from build123d import *

# Parameters (mm, degrees)
SKETCH1_R           = 35
BOSS_EXTRUDE1_DEPTH = 40
SKETCH7_R           = 5
CUT_EXTRUDE4_DEPTH  = 8
CIRPATTERN1_COUNT   = 8


with BuildPart() as part:
    # Sketch1 → Boss-Extrude1 (new body)
    with BuildSketch(Plane(origin=(0, 0, 0), x_dir=(1, 0, 0), z_dir=(0, 1, 0))):
        with Locations(Location((0, 0, 0), (0, 0, 270))):
            Circle(SKETCH1_R)
        with BuildLine():
            Line((-4, 3), (4, 3))
            ThreePointArc((4, 3), (0, -5), (-4, 3))
        make_face(mode=Mode.SUBTRACT)
    extrude(amount=BOSS_EXTRUDE1_DEPTH)

    # Sketch7 → Cut-Extrude4 (cut)
    with BuildSketch(Plane(origin=(0, 0, -35), x_dir=(-1, 0, 0), z_dir=(0, 0, -1))):
        with Locations((0, 20)):
            Circle(SKETCH7_R)
    cut_extrude4 = extrude(amount=-CUT_EXTRUDE4_DEPTH, mode=Mode.SUBTRACT)

    # CirPattern1: Cut-Extrude4 ×8 about axis
    cirpattern1_axis = Axis((0, 0, 0), (0, 1, 0))
    for i in range(1, CIRPATTERN1_COUNT):
        add(cut_extrude4.rotate(cirpattern1_axis, i * 360 / CIRPATTERN1_COUNT), mode=Mode.SUBTRACT)


solid = part.part
Here's how the part is built. I have some questions about the finished solid (model axes, mm). A direction names the side the tool comes from. Coordinates: 2 decimals unless noted, no trailing zeros. Write each loop counter-clockwise with the first axis right and the second up, starting at its lowest first coordinate (ties: lowest second). Pieces come first, ordered by that corner, then holes.
Item 1: I want a section at D-D on x = -12. Write out the boundary of the cut face in (y, z).
Item 2: I want a section at A-A on z = 0. Write out the boundary of the cut face in (x, y).
Item 3: On a 3-axis mill with a long thin cutter (end or side, diameter ignored), from which of +Z, -Z, +X, -X, +Y, -Y can I reach the whole of each face in a straight line? I mean faces 4 (the flat face through (-19.042, 20.07, -19.141)), 5 (the cylindrical face through (31.06, 15.12, 1.08)), 6 (the cylindrical face through (-1.08, 15.12, 31.06)), 7 (the flat face through (0, 20, -27)), 8 (the cylindrical face through (-31.06, 15.12, -1.08)). Say none if no direction works.
Item 4: I want a section at B-B on x = 0. Write out the boundary of the cut face in (y, z).
Item 5: If we mould it in two halves opening along Y, with no side actions, what happens to faces 1 (the flat face through (-7, 40, 0)), 2 (the flat face through (-7, 0, 0)), 3 (the flat face through (-27, 20, 0))? For each: +Y half, -Y half, draft (parallel to the pull), parting line (faces both ways), or undercut.
Item 6: If I drill on line 1 (Y direction, x = 0, z = -33); line 2 (X direction, y = 24.5, z = -29); line 3 (Z direction, x = 30.5, y = 16.5), over which ranges is the centre line in solid material (lowest first)?
Item 7: Will these pins go through, and if not, where does the flat tip stop? pin 1 (13 mm diameter, centred on x = 0, y = 20, fed in from -Z); pin 2 (8 mm diameter, centred on y = 30.5, z = 17, fed in from -X); pin 3 (3 mm diameter, centred on y = 20.5, z = 0, fed in from +X); pin 4 (5 mm diameter, centred on x = -0.5, y = 22, fed in from -Z).
Findings below:
1. outline: (0, -32.88) - (40, -32.88) - (40, 32.88) - (0, 32.88) - close
2. outline: (-35, 0) - (-5, 0) - (-5, 40) - (-35, 40) - (-35, 25) - (-27, 25) - (-27, 15) - (-35, 15) - close; (5, 0) - (35, 0) - (35, 15) - (27, 15) - (27, 25) - (35, 25) - (35, 40) - (5, 40) - close
3. face 4: none
3. face 5: +X
3. face 6: +Z
3. face 7: -Z
3. face 8: -X
4. outline: (0, -35) - (15, -35) - (15, -27) - (25, -27) - (25, -35) - (40, -35) - (40, -3) - (0, -3) - close; (0, 5) - (40, 5) - (40, 35) - (25, 35) - (25, 27) - (15, 27) - (15, 35) - (0, 35) - close
5. face 1: +Y half
5. face 2: -Y half
5. face 3: undercut
6. line 1: y = 0 to 15, 25 to 40
6. line 2: x = -19.6 to -2.18, 2.18 to 19.6
6. line 3: z = -17.17 to -3.57, 3.57 to 17.17
7. pin 1: stops at z = -35
7. pin 2: stops at x = -32.5
7. pin 3: stops at x = 27
7. pin 4: stops at z = -27
